from build123d import *

# Parameters (mm, degrees)
F0_W     = 40
F0_H     = 40
F1_DEPTH = 160
F2_R     = 15
F3_DEPTH = 100
F4_W     = 33
F4_H     = 33
F5_DEPTH = 60
F6_R     = 1


with BuildPart() as f1:
    # F0 (on Front) → F1 (new body)
    with BuildSketch(Plane.XZ):
        Rectangle(F0_W, F0_H)
    extrude(amount=F1_DEPTH)

    # F2 (on face) → F3 (cut)
    with BuildSketch(Plane.XZ.offset(160)):
        Circle(F2_R)
    extrude(amount=-F3_DEPTH, mode=Mode.SUBTRACT)

    # F4 (on face) → F5 (cut)
    with BuildSketch(Plane(origin=(0, 0, 0), x_dir=(-1, 0, 0), z_dir=(0, 1, 0))):
        Rectangle(F4_W, F4_H)
    extrude(amount=-F5_DEPTH, mode=Mode.SUBTRACT)

    # F6
    f6_edges = [f1.edges().sort_by_distance(p)[0] for p in [
        (20, -80, 20),
        (-20, -80, 20),
        (20, -80, -20),
        (-20, -80, -20),
    ]]
    fillet(f6_edges, radius=F6_R)


solid = f1.part
Source: CAD feature listing. Evaluate the final solid. Frame: model axes, mm. A direction names the side the tool comes from. Give positions to 0.01 mm unless a question says otherwise; leave off trailing zeros. Loops run counter-clockwise (first coordinate to the right, second up) from the corner with the lowest first, then second, coordinate; pieces in that order, holes last. Notation, with made-up numbers: (21.5, 87.5) -> (50.5, 87.5) arc R16 cw to (50.5, 94.5) -> close; hole circle Ø2 at (-27, -11). An arc over 180 degrees is marked (long way). Use a Markdown table: item, result. Add a question column.
1) Section query B-B, the plane x = 12. Return the cut outline in (y, z), then the cut area to 3 significant figures.
2) First-contact query: pin 1 (16.5 mm diameter, centred on x = -3.5, z = -5, fed in from +Y). Flat tip, straight axial feed; report the tip coordinate or a pass-through.
3) Reachability of faces 5 (the face through (0, -30, 16.5)), 6 (the face through (-14.985, -110.7, 0.66)) from +Z, -Z, +X, -X, +Y, -Y: full face, straight path, thin tool, end or side. Return the list, or none.
4) Pull-direction query (Z, two-part tool) for faces 1 (the face through (20, -79, 0)), 2 (the face through (-15, -60, 4)), 3 (the face through (-16.5, -30, 0)), 4 (the face through (0, -79, 20)); classes: +Z half, -Z half, draft (parallel to the pull), parting line (faces both ways), or undercut.
5) Line query: line 1 along Z through (x, y) = (-0.5, -94); line 2 along Z through (x, y) = (-11, -27.5). Output: solid intervals per line, ascending. Write a range as [from, to].
6) Section query A-A, the plane z = 0. Return the cut outline in (x, y).
7) Section query C-C, the plane y = -41. Return the cut outline in (x, z).
Numbers:
| question | item | result |
|---|---|---|
| 1 | outline | (-160, -20) -> (0, -20) -> (0, -16.5) -> (-60, -16.5) -> (-60, -9) -> (-160, -9) -> close; (-160, 9) -> (-60, 9) -> (-60, 16.5) -> (0, 16.5) -> (0, 20) -> (-160, 20) -> close |
| 1 | area | 2,620 mm2 |
| 2 | pin 1 | passes through |
| 3 | face 5 | +Y |
| 3 | face 6 | +Y, -Y |
| 4 | face 1 | draft |
| 4 | face 2 | undercut |
| 4 | face 3 | undercut |
| 4 | face 4 | +Z half |
| 5 | line 1 | z = [-20, -14.99], [14.99, 20] |
| 5 | line 2 | z = [-20, -16.5], [16.5, 20] |
| 6 | outline | (-20, -160) -> (-15, -160) -> (-15, -60) -> (-16.5, -60) -> (-16.5, 0) -> (-20, 0) -> close; (15, -160) -> (20, -160) -> (20, 0) -> (16.5, 0) -> (16.5, -60) -> (15, -60) -> close |
| 7 | outline | (-20, -19) arc R1 ccw to (-19, -20) -> (19, -20) arc R1 ccw to (20, -19) -> (20, 19) arc R1 ccw to (19, 20) -> (-19, 20) arc R1 ccw to (-20, 19) -> close; hole (-16.5, -16.5) -> (16.5, -16.5) -> (16.5, 16.5) -> (-16.5, 16.5) -> close |
